Can you work these out from the model? Positions are in its coordinate system, mm. Face numbers are marked on the shaded views. A direction names the side the tool comes from. Coordinates: 2 decimals unless noted, no trailing zeros. Order: outer loops, then holes, each group sorted by start corner. A loop starts at its lowest first (then second) coordinate and runs counter-clockwise, first axis right, second up. Notation, with made-up numbers: (58.5, 60) - (93.5, 60) arc R13 ccw to (93.5, 85) - close; hole circle Ø10 at (-23.5, 40.5). An arc over 180 degrees is marked (long way). Use a Markdown table: item, result. Add a question column.
(1) We'd pull the mould along Z, two halves only. Please class the marked faces 1, 2 and 3: pulls with the +Z half, pulls with the -Z half, needs draft (parallel to the pull), parting line crosses it, or undercut.
(2) If I drill on L1, parallel to Z at x = -10, y = 4; L2, parallel to Y at x = -23.5, z = 28.5; L3, parallel to X at y = -15, z = 13.5, over which ranges is the centre line in solid material (lowest first)? Write a range as [from, to].
(3) I want a section at B-B (x = -23.5). List the corners of the cut face in (y, z) for me.
(4) I want a section at A-A (z = -36). List the corners of the cut face in (x, y) for me, and give its area (3 significant figures).
(5) For pin 1 Ø6 at (x, y) = (-33.5, -14.5) entering from +Z; pin 2 Ø2.5 at (x, y) = (43.5, -19) entering from -Z; pin 3 Ø5 at (x, z) = (9, 25.5) entering from +Y; pin 4 Ø8 at (x, z) = (29, -16) entering from +Y, each with a flat end and sliding along its axis, tell me the tip position at first contact or that it passes through.
(6) On a 3-axis mill with a long thin cutter (end or side, diameter ignored), from which of +Z, -Z, +X, -X, +Y, -Y can I reach the whole of each face in a straight line? I mean the marked faces 4 and 5. Say none if no direction works.
(7) I want a section at D-D (x = -43). List the corners of the cut face in (y, z) for me, and give its area (3 significant figures).
(8) I want a section at C-C (y = -8). List the corners of the cut face in (x, z) for me.
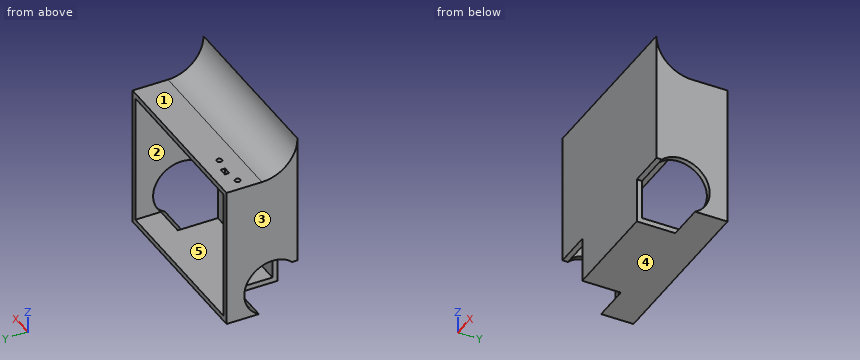
```python
from build123d import *

# Parameters (mm, degrees)
ESBO_O1_W                  = 100
ESBO_O1_H                  = 100
RESSALTO_EXTRUS_O1_DEPTH   = 20
CORTE_EXTRUS_O1_DEPTH      = 74.484692283
CORTE_EXTRUS_O1_DEPTH_BACK = 74.484692283
ESBO_O2_R                  = 20
ESBO_O3_W                  = 94
ESBO_O3_H                  = 74
CORTE_EXTRUS_O2_DEPTH      = 74.484692283
ESBO_O5_W                  = 94
ESBO_O5_H                  = 74
CORTE_EXTRUS_O3_DEPTH      = 17
CORTE_EXTRUS_O4_START      = 50
ESBO_O6_R                  = 16
CORTE_EXTRUS_O4_DEPTH      = 21
CORTE_EXTRUS_O5_START      = -29
ESBO_O6_4_R                = 16
CORTE_EXTRUS_O5_DEPTH      = 21
ESBO_O7_W                  = 21
ESBO_O7_H                  = 3.872983347
CORTE_EXTRUS_O6_DEPTH      = 21
ESBO_O8_R                  = 1.5
ESBO_O8_W                  = 4.5
ESBO_O8_H                  = 2.5
CORTE_EXTRUS_O8_DEPTH      = 74.484692283


with BuildPart() as part:
    # Esboço1 → Ressalto-extrusão1 (new, symmetric)
    with BuildSketch(Plane(origin=(0, 0, 0), x_dir=(1, 0, 0), z_dir=(0, 1, 0))):
        Rectangle(ESBO_O1_W, ESBO_O1_H)
    extrude(amount=RESSALTO_EXTRUS_O1_DEPTH, both=True)

    # Esboço2 → Corte-extrusão1 (cut, two sides: drawn at the far end of the back side and taken through both)
    with BuildSketch(Plane(origin=(0, 0, 0), x_dir=(0, 0, -1), z_dir=(1, 0, 0)).offset(-CORTE_EXTRUS_O1_DEPTH_BACK)):
        with BuildLine():
            Line((-30, 20), (-50, 20))
            ThreePointArc((-50, 20), (-35.857864376, 14.142135624), (-30, 0))
            Line((-30, 0), (-30, 20))
        make_face()
        with Locations((-50, 0)):
            Circle(ESBO_O2_R)
    extrude(amount=CORTE_EXTRUS_O1_DEPTH + CORTE_EXTRUS_O1_DEPTH_BACK, mode=Mode.SUBTRACT)

    # Esboço3 → Corte-extrusão2 (cut, through all)
    with BuildSketch(Plane(origin=(0, 0, 0), x_dir=(1, 0, 0), z_dir=(0, 1, 0))):
        with Locations((0, 10)):
            Rectangle(ESBO_O3_W, ESBO_O3_H)
    extrude(amount=CORTE_EXTRUS_O2_DEPTH, mode=Mode.SUBTRACT)

    # Esboço5 → Corte-extrusão3 (cut)
    with BuildSketch(Plane(origin=(0, 0, 0), x_dir=(1, 0, 0), z_dir=(0, 1, 0))):
        with Locations((0, 10)):
            Rectangle(ESBO_O5_W, ESBO_O5_H)
    extrude(amount=-CORTE_EXTRUS_O3_DEPTH, mode=Mode.SUBTRACT)

    # Esboço6 → Corte-extrusão4 (cut)
    with BuildSketch(Plane(origin=(0, 0, 0), x_dir=(0, 0, -1), z_dir=(1, 0, 0)).offset(CORTE_EXTRUS_O4_START)):
        with Locations((36, -6)):
            Circle(ESBO_O6_R)
        with BuildLine():
            ThreePointArc((52, -6), (47.313708499, -17.313708499), (36, -22))
            Line((36, -22), (52, -22))
            Line((52, -22), (52, -6))
        make_face()
    extrude(amount=-CORTE_EXTRUS_O4_DEPTH, mode=Mode.SUBTRACT)

    # Esboço6<4> → Corte-extrusão5 (cut)
    with BuildSketch(Plane(origin=(0, 0, 0), x_dir=(0, 0, -1), z_dir=(1, 0, 0)).offset(CORTE_EXTRUS_O5_START)):
        with BuildLine():
            ThreePointArc((52, -6), (47.313708499, -17.313708499), (36, -22))
            Line((36, -22), (52, -22))
            Line((52, -22), (52, -6))
        make_face()
        with Locations((36, -6)):
            Circle(ESBO_O6_4_R)
    extrude(amount=-CORTE_EXTRUS_O5_DEPTH, mode=Mode.SUBTRACT)

    # Esboço7 → Corte-extrusão6 (cut)
    with BuildSketch(Plane(origin=(0, 0, 0), x_dir=(1, 0, 0), z_dir=(0, 1, 0))):
        with Locations((-39.5, 26.317541635)):
            Rectangle(ESBO_O7_W, ESBO_O7_H)
        with Locations((39.5, 26.317541635)):
            Rectangle(ESBO_O7_W, ESBO_O7_H)
    extrude(amount=-CORTE_EXTRUS_O6_DEPTH, mode=Mode.SUBTRACT)

    # Esboço8 → Corte-extrusão8 (cut, through all)
    with BuildSketch(Plane.XY):
        with Locations(Location((-43, 10, 0), (0, 0, 180))):
            Circle(ESBO_O8_R)
        with Locations(Location((-23.5, 10, 0), (0, 0, 180))):
            Circle(ESBO_O8_R)
        with Locations((-33.25, 12)):
            Rectangle(ESBO_O8_W, ESBO_O8_H)
    extrude(amount=CORTE_EXTRUS_O8_DEPTH, mode=Mode.SUBTRACT)


solid = part.part
```
Answers follow:
| question | item | result |
|---|---|---|
| 1 | face 1 | pulls with the +Z half |
| 1 | face 2 | undercut |
| 1 | face 3 | needs draft |
| 2 | L1 | z = [-50, -47], [27, 30] |
| 2 | L2 | y = [-20, 8.5], [11.5, 20] |
| 2 | L3 | x = [-50, -47], [47, 50] |
| 3 | outline | (-20, -50) - (20, -50) - (20, -47) - (-17, -47) - (-17, 27) - (8.5, 27) - (8.5, 30) - (0, 30) arc R20 cw to (-20, 50) - close; (11.5, 27) - (20, 27) - (20, 30) - (11.5, 30) - close |
| 4 | outline | (-50, 10) - (-47, 10) - (-47, 20) - (-50, 20) - close; (-29, -20) - (29, -20) - (29, -17) - (-29, -17) - close; (47, 10) - (50, 10) - (50, 20) - (47, 20) - close |
| 4 | area | 234 mm² |
| 5 | pin 1 | stops at z = 40.32 |
| 5 | pin 2 | stops at z = -24.38 |
| 5 | pin 3 | stops at y = 20 |
| 5 | pin 4 | stops at y = -17 |
| 6 | face 4 | -Z, +X, -X, +Y, -Y |
| 6 | face 5 | +Y |
| 7 | outline | (-20, -24.38) - (-17, -24.38) - (-17, 27) - (8.5, 27) - (8.5, 30) - (0, 30) arc R20 cw to (-20, 50) - close; (1.75, -50) - (20, -50) - (20, -47) - (5.62, -47) arc R16 cw to start; (11.5, 27) - (20, 27) - (20, 30) - (11.5, 30) - close |
| 7 | area | 399 mm² |
| 8 | outline | (-50, -20.13) - (-47, -20.13) - (-47, 27) - (47, 27) - (47, -20.13) - (50, -20.13) - (50, 31.67) - (-50, 31.67) - close; (-29, -50) - (29, -50) - (29, -47) - (-29, -47) - close |
